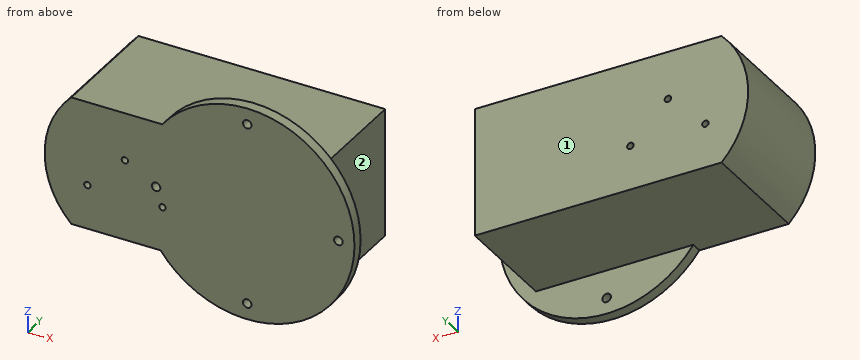
from build123d import *

# Parameters (mm, degrees)
SKETCH1_R                = 50
BOSS_EXTRUDE1_DEPTH      = 5
BOSS_EXTRUDE2_DEPTH      = 50
BOSS_EXTRUDE2_DEPTH_BACK = 5
SKETCH3_R                = 2
CUT_EXTRUDE1_DEPTH       = 50
BOSS_EXTRUDE3_DEPTH      = 55
SKETCH5_R                = 1.5
CUT_EXTRUDE2_DEPTH       = 55


with BuildPart() as part:
    # Sketch1 → Boss-Extrude1 (new body)
    with BuildSketch(Plane(origin=(0, 0, 0), x_dir=(1, 0, 0), z_dir=(0, 1, 0))):
        with Locations(Location((0, 0, 0), (0, 0, 270))):
            Circle(SKETCH1_R)
    extrude(amount=BOSS_EXTRUDE1_DEPTH)

    # Sketch2 → Boss-Extrude2 (add, two sides: drawn at the far end of the back side and taken through both)
    with BuildSketch(Plane(origin=(0, 5, 0), x_dir=(1, 0, 0), z_dir=(0, 1, 0)).offset(-BOSS_EXTRUDE2_DEPTH_BACK)):
        with BuildLine():
            ThreePointArc((-40.394880662, 29.46614356), (-49.995546188, -0.667353994), (-39.593984529, -30.53385644))
            Line((-39.593984529, -30.53385644), (33, -30.53385644))
            Line((33, -30.53385644), (33, 29.46614356))
            Line((33, 29.46614356), (-40.394880662, 29.46614356))
        make_face()
        with BuildLine():
            Line((-82, 29.46614356), (-82, -30.53385644))
            Line((-82, -30.53385644), (-39.593984529, -30.53385644))
            ThreePointArc((-39.593984529, -30.53385644), (-49.995546188, -0.667353994), (-40.394880662, 29.46614356))
            Line((-40.394880662, 29.46614356), (-82, 29.46614356))
        make_face()
    extrude(amount=BOSS_EXTRUDE2_DEPTH + BOSS_EXTRUDE2_DEPTH_BACK)

    # Sketch3 → Cut-Extrude1 (cut)
    with BuildSketch(Plane(origin=(0, 5, 0), x_dir=(1, 0, 0), z_dir=(0, 1, 0))):
        with Locations(Location((0, -42.5, 0), (0, 0, 270))):
            Circle(SKETCH3_R)
        with Locations(Location((-42.5, 0, 0), (0, 0, 270))):
            Circle(SKETCH3_R)
        with Locations(Location((0, 42.5, 0), (0, 0, 270))):
            Circle(SKETCH3_R)
        with Locations(Location((42.5, 0, 0), (0, 0, 270))):
            Circle(SKETCH3_R)
    extrude(amount=-CUT_EXTRUDE1_DEPTH, mode=Mode.SUBTRACT)

    # Sketch4 → Boss-Extrude3 (add)
    with BuildSketch(Plane(origin=(0, 55, 0), x_dir=(1, 0, 0), z_dir=(0, 1, 0))):
        with BuildLine():
            Line((-82, 29.46614356), (-82, -30.53385644))
            ThreePointArc((-82, -30.53385644), (-94.426406871, -0.53385644), (-82, 29.46614356))
        make_face()
    extrude(amount=-BOSS_EXTRUDE3_DEPTH)

    # Sketch5 → Cut-Extrude2 (cut)
    with BuildSketch(Plane(origin=(0, 55, 0), x_dir=(1, 0, 0), z_dir=(0, 1, 0))):
        with Locations(Location((-74.5, 8.768970361, 0), (0, 0, 270))):
            Circle(SKETCH5_R)
        with Locations(Location((-39.5, 8.768970361, 0), (0, 0, 270))):
            Circle(SKETCH5_R)
        with Locations(Location((-57, -8.231029639, 0), (0, 0, 270))):
            Circle(SKETCH5_R)
    extrude(amount=-CUT_EXTRUDE2_DEPTH, mode=Mode.SUBTRACT)


solid = part.part
Verification items for the finished model (mm, model axes). Face numbers are marked on the shaded views. A direction names the side the tool comes from. Give positions to 0.01 mm unless a question says otherwise; leave off trailing zeros. Write each loop counter-clockwise with the first axis right and the second up, starting at its lowest first coordinate (ties: lowest second). Pieces come first, ordered by that corner, then holes. Notation, with made-up numbers: M 45,-7.5 L 72,-7.5 A20 cw 72,2.5 Z; hole C 64.5,8 d7. An arc over 180 degrees is marked long. Write item = value, one per line.
(1) Material ranges on line 1 (X direction, y = 1, z = 0); line 2 (Z direction, x = -74.5, y = 25.5); line 3 (Z direction, x = -23, y = 49.5), recorded low to high.
Found:
line_1 = -94.42 to -44.5, -40.5 to 40.5, 44.5 to 50
line_2 = -29.47 to -10.27, -7.27 to 30.53
line_3 = -29.47 to 30.53
(2) Go/stop test with flat-tipped pins: pin 1 Ø8 at (y, z) = (8, 24) entering from +X; pin 2 Ø2.5 at (x, z) = (-57, 8.23) entering from -Y (3 decimals); pin 3 Ø2 at (y, z) = (30, -20) entering from +X; pin 4 Ø5 at (x, z) = (0, 42.5) entering from +Y. Record where each tip stops, or that it passes through.
Found:
pin_1 = 45.21
pin_2 = through
pin_3 = 33
pin_4 = 5
(3) Sectioned sample at B-B (z = 43). Record the cut outline in (x, y), then the cut area to 3 significant figures.
Found:
outline = M -25.51,0 L -1.94,0 L -1.94,5 L -25.51,5 Z; M 1.94,0 L 25.51,0 L 25.51,5 L 1.94,5 Z
area = 236 mm2
(4) Sectioned sample at C-C (x = -42.5). Record the cut outline in (y, z).
Found:
outline = M 0,-29.47 L 55,-29.47 L 55,30.53 L 0,30.53 L 0,2 L 5,2 L 5,-2 L 0,-2 Z
(5) Sectioned sample at D-D (z = -42). Record the cut outline in (x, y), then the cut area to 3 significant figures.
Found:
outline = M -27.13,0 L -1.94,0 L -1.94,5 L -27.13,5 Z; M 1.94,0 L 27.13,0 L 27.13,5 L 1.94,5 Z
area = 252 mm2
(6) Sectioned sample at A-A (y = 37.5). Record the cut outline in (x, z).
Found:
outline = M -82,-29.47 L 33,-29.47 L 33,30.53 L -82,30.53 A42.43 ccw Z; hole C -74.5,-8.77 d3; hole C -57,8.23 d3; hole C -39.5,-8.77 d3
(7) Access from +Z, -Z, +X, -X, +Y, -Y to the whole of each face (thin tool, end or side, straight path). Record for the marked faces 1 and 2.
Found:
face_1 = +Z, -Z, +X, -X, +Y
face_2 = +Z, -Z, +X, +Y
